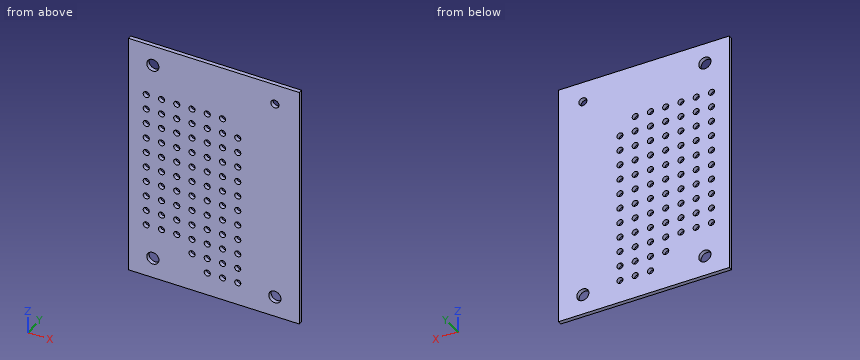
from build123d import *

# Parameters (mm, degrees)
F0_W     = 84
F0_H     = 120
F0_R     = 3
F0_R_2   = 2
F1_DEPTH = 2
F2_R     = 1.5
F3_DEPTH = 2.001
F4_R     = 1.5
F5_DEPTH = 2.001


with BuildPart() as f1:
    # F0 (on Front) → F1 (new body)
    with BuildSketch(Plane.XZ):
        Rectangle(F0_W, F0_H)
        with Locations((-30, -50)):
            Circle(F0_R, mode=Mode.SUBTRACT)
        with Locations((30, -50)):
            Circle(F0_R, mode=Mode.SUBTRACT)
        with Locations((-30, 50)):
            Circle(F0_R, mode=Mode.SUBTRACT)
        with Locations((30, 50)):
            Circle(F0_R_2, mode=Mode.SUBTRACT)
    extrude(amount=F1_DEPTH)

    # F2 (on face) → F3 (cut, through all)
    with BuildSketch(Plane.XZ.offset(2)):
        with Locations((-33.25, 33.75)):
            Circle(F2_R)
        with Locations((-33.25, 26.25)):
            Circle(F2_R)
        with Locations((-33.25, 18.75)):
            Circle(F2_R)
        with Locations((-33.25, 11.25)):
            Circle(F2_R)
        with Locations((-33.25, 3.75)):
            Circle(F2_R)
        with Locations((-33.25, -3.75)):
            Circle(F2_R)
        with Locations((-33.25, -11.25)):
            Circle(F2_R)
        with Locations((-33.25, -18.75)):
            Circle(F2_R)
        with Locations((-33.25, -26.25)):
            Circle(F2_R)
        with Locations((-33.25, -33.75)):
            Circle(F2_R)
        with Locations((-25.75, 33.75)):
            Circle(F2_R)
        with Locations((-25.75, 26.25)):
            Circle(F2_R)
        with Locations((-25.75, 18.75)):
            Circle(F2_R)
        with Locations((-25.75, 11.25)):
            Circle(F2_R)
        with Locations((-25.75, 3.75)):
            Circle(F2_R)
        with Locations((-25.75, -3.75)):
            Circle(F2_R)
        with Locations((-25.75, -11.25)):
            Circle(F2_R)
        with Locations((-25.75, -18.75)):
            Circle(F2_R)
        with Locations((-25.75, -26.25)):
            Circle(F2_R)
        with Locations((-25.75, -33.75)):
            Circle(F2_R)
        with Locations((-18.25, 33.75)):
            Circle(F2_R)
        with Locations((-18.25, 26.25)):
            Circle(F2_R)
        with Locations((-18.25, 18.75)):
            Circle(F2_R)
        with Locations((-18.25, 11.25)):
            Circle(F2_R)
        with Locations((-18.25, 3.75)):
            Circle(F2_R)
        with Locations((-18.25, -3.75)):
            Circle(F2_R)
        with Locations((-18.25, -11.25)):
            Circle(F2_R)
        with Locations((-18.25, -18.75)):
            Circle(F2_R)
        with Locations((-18.25, -26.25)):
            Circle(F2_R)
        with Locations((-18.25, -33.75)):
            Circle(F2_R)
        with Locations((-10.75, 33.75)):
            Circle(F2_R)
        with Locations((-10.75, 26.25)):
            Circle(F2_R)
        with Locations((-10.75, 18.75)):
            Circle(F2_R)
        with Locations((-10.75, 11.25)):
            Circle(F2_R)
        with Locations((-10.75, 3.75)):
            Circle(F2_R)
        with Locations((-10.75, -3.75)):
            Circle(F2_R)
        with Locations((-10.75, -11.25)):
            Circle(F2_R)
        with Locations((-10.75, -18.75)):
            Circle(F2_R)
        with Locations((-10.75, -26.25)):
            Circle(F2_R)
        with Locations((-10.75, -33.75)):
            Circle(F2_R)
        with Locations((-3.25, 33.75)):
            Circle(F2_R)
        with Locations((-3.25, 26.25)):
            Circle(F2_R)
        with Locations((-3.25, 18.75)):
            Circle(F2_R)
        with Locations((-3.25, 11.25)):
            Circle(F2_R)
        with Locations((-3.25, 3.75)):
            Circle(F2_R)
        with Locations((-3.25, -3.75)):
            Circle(F2_R)
        with Locations((-3.25, -11.25)):
            Circle(F2_R)
        with Locations((-3.25, -18.75)):
            Circle(F2_R)
        with Locations((-3.25, -26.25)):
            Circle(F2_R)
        with Locations((-3.25, -33.75)):
            Circle(F2_R)
        with Locations((4.25, 33.75)):
            Circle(F2_R)
        with Locations((4.25, 26.25)):
            Circle(F2_R)
        with Locations((4.25, 18.75)):
            Circle(F2_R)
        with Locations((4.25, 11.25)):
            Circle(F2_R)
        with Locations((4.25, 3.75)):
            Circle(F2_R)
        with Locations((4.25, -3.75)):
            Circle(F2_R)
        with Locations((4.25, -11.25)):
            Circle(F2_R)
        with Locations((4.25, -18.75)):
            Circle(F2_R)
        with Locations((4.25, -26.25)):
            Circle(F2_R)
        with Locations((4.25, -33.75)):
            Circle(F2_R)
        with Locations((11.75, 26.25)):
            Circle(F2_R)
        with Locations((11.75, 18.75)):
            Circle(F2_R)
        with Locations((11.75, 11.25)):
            Circle(F2_R)
        with Locations((11.75, 3.75)):
            Circle(F2_R)
        with Locations((11.75, -3.75)):
            Circle(F2_R)
        with Locations((11.75, -11.25)):
            Circle(F2_R)
        with Locations((11.75, -18.75)):
            Circle(F2_R)
        with Locations((11.75, -26.25)):
            Circle(F2_R)
        with Locations((11.75, -33.75)):
            Circle(F2_R)
    extrude(amount=-F3_DEPTH, mode=Mode.SUBTRACT)

    # F4 (on face) → F5 (cut, through all)
    with BuildSketch(Plane.XZ.offset(2)):
        with BuildLine():
            ThreePointArc((13.25, -41.25), (12.81066, -40.18934), (11.75, -39.75))
            Line((11.75, -39.75), (11.75, -42.75))
            ThreePointArc((11.75, -42.75), (12.81066, -42.31066), (13.25, -41.25))
        make_face()
        with BuildLine():
            Line((11.75, -42.75), (11.75, -39.75))
            ThreePointArc((11.75, -39.75), (10.25, -41.25), (11.75, -42.75))
        make_face()
        with Locations((11.75, -48.75)):
            Circle(F4_R)
        with Locations((4.25, -41.25)):
            Circle(F4_R)
        with Locations((4.25, -48.75)):
            Circle(F4_R)
        with Locations((-3.25, -41.25)):
            Circle(F4_R)
        with Locations((-3.25, -48.75)):
            Circle(F4_R)
        with Locations((-10.75, -41.25)):
            Circle(F4_R)
    extrude(amount=-F5_DEPTH, mode=Mode.SUBTRACT)


solid = f1.part
For this review, take the finished solid that the model builds, in its own axes (mm). Round coordinates to 2 decimals unless told otherwise and drop trailing zeros. Write each loop counter-clockwise with the first axis right and the second up, starting at its lowest first coordinate (ties: lowest second). Pieces come first, ordered by that corner, then holes. Notation, with made-up numbers: (-23.75, -8) -> (24.25, -8) arc R29 ccw to (24.25, 24) -> close; hole circle Ø6 at (-35, -31.5). An arc over 180 degrees is marked (long way). Use CSV: the item, a comma, the result in double quotes.
(1) Consider section B-B, the plane x = 30. Give the boundary of the cut face in (y, z), plus the area to 3 significant figures.
Computed values:
outline,"(-2, -60) -> (0, -60) -> (0, -53) -> (-2, -53) -> close; (-2, -47) -> (0, -47) -> (0, 48) -> (-2, 48) -> close; (-2, 52) -> (0, 52) -> (0, 60) -> (-2, 60) -> close"
area,"220 mm²"
(2) Consider section C-C, the plane z = -48.75. Give the boundary of the cut face in (x, y).
Computed values:
outline,"(-42, -2) -> (-32.73, -2) -> (-32.73, 0) -> (-42, 0) -> close; (-27.27, -2) -> (-4.75, -2) -> (-4.75, 0) -> (-27.27, 0) -> close; (-1.75, -2) -> (2.75, -2) -> (2.75, 0) -> (-1.75, 0) -> close; (5.75, -2) -> (10.25, -2) -> (10.25, 0) -> (5.75, 0) -> close; (13.25, -2) -> (27.27, -2) -> (27.27, 0) -> (13.25, 0) -> close; (32.73, -2) -> (42, -2) -> (42, 0) -> (32.73, 0) -> close"
(3) Consider section A-A, the plane z = -11.25. Give the number of separate pieces and of enclosed holes in the cut face, plus the area to 3 significant figures.
Computed values:
separate pieces,"8"
enclosed holes,"0"
area,"126 mm²"
(4) To check wall thickness, follow L1, parallel to Z at x = -30, y = -1.4; L2, parallel to Z at x = 29, y = -0.5; L3, parallel to Z at x = 27.5, y = -1.15. State the ranges of each line that lie inside material, in increasing order. Write a range as [from, to].
Computed values:
L1,"[-60, -53], [-47, 47], [53, 60]"
L2,"[-60, -52.83], [-47.17, 48.27], [51.73, 60]"
L3,"[-60, -51.66], [-48.34, 60]"
